Model file for the job. Use its own axes, mm. A direction names the side the tool comes from. Give positions to 0.01 mm unless a question says otherwise; leave off trailing zeros. Order: outer loops, then holes, each group sorted by start corner. A loop starts at its lowest first (then second) coordinate and runs counter-clockwise, first axis right, second up. Notation, with made-up numbers: (5, 44.25) - (13, 44.25) arc R21 cw to (13, 73.25) - close; hole circle Ø10 at (28, -36). An arc over 180 degrees is marked (long way). Use CSV: the item, a comma, the result in double quotes. Start each with the question number.
(1) Band-saw the part on A-A, the plane x = 3.5. Give the cut face in (y, z), then the cut area to 3 significant figures.
(2) Band-saw the part on B-B, the plane x = 23.5. Give the cut face in (y, z).
(3) Drop flat-ended pins along their axis: pin 1 Ø0.9 at (y, z) = (-47.5, 37) entering from -X; pin 2 Ø5 at (x, z) = (23.5, 25) entering from +Y; pin 3 Ø1.8 at (y, z) = (-47.5, 12.5) entering from +X; pin 4 Ø3.5 at (y, z) = (-47.5, 12) entering from -X. Give the stop position or say it passes through.
(4) Band-saw the part on C-C, the plane z = 8.5. Give the cut face in (x, y).
(5) Band-saw the part on D-D, the plane x = 11.5. Give the cut face in (y, z).
(6) Probe L1, parallel to Y at x = 0.5, z = 37.5; L2, parallel to X at y = -47.5, z = 47; L3, parallel to X at y = -47.25, z = 25.5. List the from-to ranges inside material, lowest first.
(7) Pull direction X, two halves, no side cores. Call faces 1 (the cylindrical face through (26.752, -47.465, 10.357)), 2 (the flat face through (42.5, -47, 38)), 3 (the flat face through (23, -53, 19)), 4 (the flat face through (20, -50, 25)): +X half, -X half, draft (parallel to the pull), parting line (faces both ways), or undercut.
(8) Tool access for faces 5 (the cylindrical face through (47.57, -48.964, 12.825)), 6 (the flat face through (52.5, -49, 25)), 7 (the cylindrical face through (-0.57, -48.964, 37.175)): list every direction of +Z, -Z, +X, -X, +Y, -Y with a clear straight run to the whole face (end or side of a thin tool).
from build123d import *

# Parameters (mm, degrees)
ESQUISSE1_W             = 58
ESQUISSE1_H             = 8
BOSS_EXTRU_1_DEPTH      = 50
ESQUISSE2_R             = 15
ENL_V_MAT_EXTRU_1_DEPTH = 5
ESQUISSE3_R             = 1.5
ENL_V_MAT_EXTRU_2_DEPTH = 10
ESQUISSE4_R             = 1.5
ENL_V_MAT_EXTRU_3_DEPTH = 10
ESQUISSE5_R             = 1.5
ENL_V_MAT_EXTRU_4_DEPTH = 4
ESQUISSE6_R             = 1.5
ENL_V_MAT_EXTRU_5_DEPTH = 51


with BuildPart() as part:
    # Esquisse1 → Boss.-Extru.1 (new body)
    with BuildSketch(Plane.XY):
        with Locations((23.5, -49)):
            Rectangle(ESQUISSE1_W, ESQUISSE1_H)
    extrude(amount=BOSS_EXTRU_1_DEPTH)

    # Esquisse2 → Enlèv. mat.-Extru.1 (cut)
    with BuildSketch(Plane(origin=(0, -45, 0), x_dir=(-1, 0, 0), z_dir=(0, 1, 0))):
        with Locations((-23.5, 25)):
            Circle(ESQUISSE2_R)
    extrude(amount=-ENL_V_MAT_EXTRU_1_DEPTH, mode=Mode.SUBTRACT)

    # Esquisse3 → Enlèv. mat.-Extru.2 (cut)
    with BuildSketch(Plane.ZY.offset(5.5)):
        with Locations((12.5, -47.5)):
            Circle(ESQUISSE3_R)
        with Locations((37.5, -47.5)):
            Circle(ESQUISSE3_R)
    extrude(amount=-ENL_V_MAT_EXTRU_2_DEPTH, mode=Mode.SUBTRACT)

    # Esquisse4 → Enlèv. mat.-Extru.3 (cut)
    with BuildSketch(Plane(origin=(52.5, 0, 0), x_dir=(0, 0, -1), z_dir=(1, 0, 0))):
        with Locations((-37.5, -47.5)):
            Circle(ESQUISSE4_R)
        with Locations((-12.5, -47.5)):
            Circle(ESQUISSE4_R)
    extrude(amount=-ENL_V_MAT_EXTRU_3_DEPTH, mode=Mode.SUBTRACT)

    # Esquisse5 → Enlèv. mat.-Extru.4 (cut, through all)
    with BuildSketch(Plane(origin=(0, -50, 0), x_dir=(1, 0, 0), z_dir=(0, 1, 0))):
        with Locations((23.5, -25)):
            Circle(ESQUISSE5_R)
    extrude(amount=-ENL_V_MAT_EXTRU_4_DEPTH, mode=Mode.SUBTRACT)

    # Esquisse6 → Enlèv. mat.-Extru.5 (cut, through all)
    with BuildSketch(Plane(origin=(0, 0, 0), x_dir=(-1, 0, 0), z_dir=(0, 0, -1))):
        with Locations((-23.5, -47.5)):
            Circle(ESQUISSE6_R)
    extrude(amount=-ENL_V_MAT_EXTRU_5_DEPTH, mode=Mode.SUBTRACT)


solid = part.part
Answer block:
1,outline,"(-53, 0) - (-45, 0) - (-45, 50) - (-53, 50) - close; hole circle Ø3 at (-47.5, 12.5); hole circle Ø3 at (-47.5, 37.5)"
1,area,"386 mm2"
2,outline,"(-53, 0) - (-49, 0) - (-49, 10) - (-50, 10) - (-50, 23.5) - (-53, 23.5) - close; (-53, 26.5) - (-50, 26.5) - (-50, 40) - (-49, 40) - (-49, 50) - (-53, 50) - close; (-46, 0) - (-45, 0) - (-45, 10) - (-46, 10) - close; (-46, 40) - (-45, 40) - (-45, 50) - (-46, 50) - close"
3,pin 1,"stops at x = 4.5"
3,pin 2,"stops at y = -50"
3,pin 3,"stops at x = 42.5"
3,pin 4,"stops at x = -5.5"
4,outline,"(-5.5, -53) - (52.5, -53) - (52.5, -45) - (-5.5, -45) - close; hole circle Ø3 at (23.5, -47.5)"
5,outline,"(-53, 0) - (-45, 0) - (-45, 16) - (-50, 16) - (-50, 34) - (-45, 34) - (-45, 50) - (-53, 50) - close"
6,L1,"y = -53 to -49, -46 to -45"
6,L2,"x = -5.5 to 22, 25 to 52.5"
6,L3,"x = -5.5 to 8.51, 38.49 to 52.5"
7,face 1,"undercut"
7,face 2,"+X half"
7,face 3,"draft"
7,face 4,"undercut"
8,face 5,"+X"
8,face 6,"+Z, -Z, +X, +Y, -Y"
8,face 7,"-X"
